The model under review builds one solid part; all positions refer to its coordinate system, in mm. A direction names the side the tool comes from. Give positions to 0.01 mm unless a question says otherwise; leave off trailing zeros. Write each loop counter-clockwise with the first axis right and the second up, starting at its lowest first coordinate (ties: lowest second). Pieces come first, ordered by that corner, then holes. Notation, with made-up numbers: M -26.75,32 L 5.25,32 A13 cw 5.25,36 Z; hole C 58,87.25 d6. An arc over 180 degrees is marked long. Write item = value, one per line. Start each with the question number.
```python
from build123d import *

# Parameters (mm, degrees)
SKETCH1_W                = 18
SKETCH1_H                = 18
BOSS_EXTRUDE1_DEPTH      = 8
M3_TAPPED_HOLE1_D        = 2.5
F_6_0_6_DIAMETER_HOLE1_D = 6
M3_TAPPED_HOLE2_REACH    = 23.656
M3_TAPPED_HOLE2_BORE_R   = 1.25
SKETCH15_R               = 12.727922061
SKETCH15_R_2             = 9
CUT_EXTRUDE1_DEPTH       = 10
FILLET1_R                = 1


with BuildPart() as part:
    # Sketch1 → Boss-Extrude1 (new body)
    with BuildSketch(Plane.XY):
        Rectangle(SKETCH1_W, SKETCH1_H)
    extrude(amount=BOSS_EXTRUDE1_DEPTH)

    # M3 Tapped Hole1 (through all)
    with Locations(Plane.XY.offset(8)):
        with Locations((6.5, 0), (-6.5, 0)):
            Hole(M3_TAPPED_HOLE1_D / 2)

    # Ø6.0 (6) Diameter Hole1 (through all)
    with Locations(Plane(origin=(0, 0, 0), x_dir=(-1, 0, 0), z_dir=(0, 0, -1))):
        with Locations((0, 0)):
            Hole(F_6_0_6_DIAMETER_HOLE1_D / 2)

    # M3 Tapped Hole2 bore → M3 Tapped Hole2 (cut, up to next)
    with BuildSketch(Plane(origin=(0, 9, 0), x_dir=(1, 0, 0), z_dir=(0, 1, 0)), mode=Mode.PRIVATE) as m3_tapped_hole2_sk1:
        with Locations((0, -4)):
            Circle(M3_TAPPED_HOLE2_BORE_R)
    m3_tapped_hole2_tool1 = extrude(m3_tapped_hole2_sk1.sketch, amount=-M3_TAPPED_HOLE2_REACH, mode=Mode.PRIVATE) & part.part
    add(m3_tapped_hole2_tool1.solids().sort_by_distance((0, 9, 4))[0], mode=Mode.SUBTRACT)

    # Sketch15 → Cut-Extrude1 (cut)
    with BuildSketch(Plane.XY.offset(8)):
        Circle(SKETCH15_R)
        Circle(SKETCH15_R_2, mode=Mode.SUBTRACT)
    extrude(amount=-CUT_EXTRUDE1_DEPTH, mode=Mode.SUBTRACT)

    # Fillet1
    fillet1_edges = [part.edges().sort_by_distance(p)[0] for p in [
        (-9, 0, 0),
        (-9, 0, 8),
    ]]
    fillet(fillet1_edges, radius=FILLET1_R)


solid = part.part
```
Item 1: We need section B-B, the plane y = 0. Write out the cut boundary in (x, z).
Item 2: The part is to be moulded in two halves that separate along Y. For faces 1 (the flat face through (3.4, 0.1, 0)), 2 (the cylindrical face through (-5.25, 0.05, 3.94)), 3 (the cylindrical face through (-1.951, -8.786, 4.042)), say which applies: released by +Y, released by -Y, zero draft, split by the parting line, or undercut.
Item 3: To check wall thickness, follow probe 1 along Z at (x, y) = (0, 7.75); probe 2 along Y at (x, z) = (6.5, 4.75); probe 3 along Y at (x, z) = (0.25, 1.5). State the ranges of each line that lie inside material, in increasing order. Write a range as [from, to].
Item 4: We need section C-C, the plane z = 4. Write out the cut boundary in (x, y), and give its area (3 significant figures).
Item 5: We need section A-A, the plane x = 0. Write out the cut boundary in (y, z), and give its area (3 significant figures).
Item 6: Clearance check with a flat-ended pin moving along its axis: P1, Ø2, axis at y = -5.5, z = 3.5, coming from the -X side. State where the tip first meets the part, or that it passes through.
Item 7: For faces 4 (the cylindrical face through (-0.27, 5.91, 5.22)), 5 (the cylindrical face through (7.75, 0.05, 3.94)), list the 3-axis set-ups (+Z, -Z, +X, -X, +Y, -Y) from which the entire face can be reached by the end or side of a thin tool; tool diameter is ignored.
Item 8: We need section D-D, the plane z = 6.25. Write out the cut boundary in (x, y).
Worked out:
q1.outline = M -9,1 A1 ccw -8,0 L -7.75,0 L -7.75,8 L -8,8 A1 ccw -9,7 Z; M -5.25,0 L -3,0 L -3,8 L -5.25,8 Z; M 3,0 L 5.25,0 L 5.25,8 L 3,8 Z; M 7.75,0 L 8,0 A1 ccw 9,1 L 9,7 A1 ccw 8,8 L 7.75,8 Z
q2.face_1 = zero draft
q2.face_2 = undercut
q2.face_3 = split by the parting line
q3.probe_1 = [0, 2.75], [5.25, 8]
q3.probe_2 = [-6.22, -1.25], [1.25, 6.22]
q3.probe_3 = [-9, -2.99], [2.99, 9]
q4.outline = M -1.25,2.73 L -1.25,8.91 A9 ccw long 1.25,8.91 L 1.25,2.73 A3 cw long Z; hole C -6.5,0 d2.5; hole C 6.5,0 d2.5
q4.area = 201 mm²
q5.outline = M -9,1 A1 ccw -8,0 L -3,0 L -3,8 L -8,8 A1 ccw -9,7 Z; M 3,0 L 8,0 A1 ccw 9,1 L 9,2.75 L 3,2.75 Z; M 3,5.25 L 9,5.25 L 9,7 A1 ccw 8,8 L 3,8 Z
q5.area = 80.1 mm²
q6.P1 = -7.79
q7.face_4 = +Y
q7.face_5 = +Z, -Z
q8.outline = C 0,0 d18; hole C -6.5,0 d2.5; hole C 0,0 d6; hole C 6.5,0 d2.5
